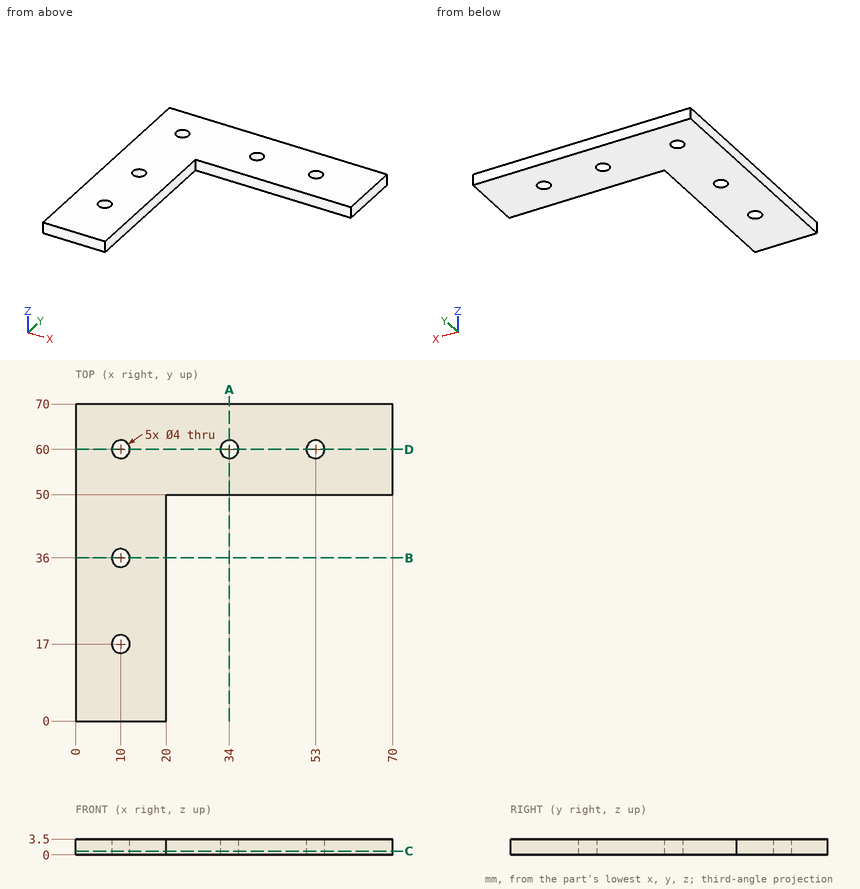
Geometry: see drawing. Coordinates: mm, zero at the bounding-box minimum. Give positions to 0.01 mm unless a question says otherwise; leave off trailing zeros. Order: outer loops, then holes, each group sorted by start corner. A loop starts at its lowest first (then second) coordinate and runs counter-clockwise, first axis right, second up. Notation, with made-up numbers: M 87.25,45 L 132.25,45 A12 cw 132.25,58 Z; hole C 17,20 d1. An arc over 180 degrees is marked long. Answer as a JSON object with one key per item and string values.
1. Cut plane C-C, the plane z = 0.85. Output: boundary loops of the cut face in (x, y).
Result sheet:
{"outline": "M 0,0 L 20,0 L 20,50 L 70,50 L 70,70 L 0,70 Z; hole C 10,17 d4; hole C 10,36 d4; hole C 10,60 d4; hole C 34,60 d4; hole C 53,60 d4"}
2. First-contact query: P1, Ø1, axis at x = 33, z = 2, coming from the -Y side. Flat tip, straight axial feed; report the tip coordinate or a pass-through.
Result sheet:
{"P1": "y = 50"}
3. Cut plane B-B, the plane y = 36. Output: boundary loops of the cut face in (x, z), and give its area (3 significant figures).
Result sheet:
{"outline": "M 0,0 L 8,0 L 8,3.5 L 0,3.5 Z; M 12,0 L 20,0 L 20,3.5 L 12,3.5 Z", "area": "56.0 mm²"}
4. Cut plane A-A, the plane x = 34. Output: boundary loops of the cut face in (y, z), and give its area (3 significant figures).
Result sheet:
{"outline": "M 50,0 L 58,0 L 58,3.5 L 50,3.5 Z; M 62,0 L 70,0 L 70,3.5 L 62,3.5 Z", "area": "56.0 mm²"}
5. Cut plane D-D, the plane y = 60. Output: boundary loops of the cut face in (x, z).
Result sheet:
{"outline": "M 0,0 L 8,0 L 8,3.5 L 0,3.5 Z; M 12,0 L 32,0 L 32,3.5 L 12,3.5 Z; M 36,0 L 51,0 L 51,3.5 L 36,3.5 Z; M 55,0 L 70,0 L 70,3.5 L 55,3.5 Z"}
6. Ray query, line 1 (Y direction, x = 10, z = 1.35); line 2 (Y direction, x = 45.5, z = 1.5); line 3 (X direction, y = 6, z = 1). Return the intervals inside material, ascending. Write a range as [from, to].
Result sheet:
{"line 1": "[0, 15], [19, 34], [38, 58], [62, 70]", "line 2": "[50, 70]", "line 3": "[0, 20]"}
